Read the model definition and answer for the solid it produces. Units are mm, in the model's axes. Coordinates: 2 decimals unless noted, no trailing zeros. Loops run counter-clockwise (first coordinate to the right, second up) from the corner with the lowest first, then second, coordinate; pieces in that order, holes last. Notation, with made-up numbers: (80.25, 54.25) -> (133.25, 54.25) arc R17 cw to (133.25, 63.25) -> close; hole circle Ø11 at (-29, 83). An arc over 180 degrees is marked (long way). Answer as a JSON object with one key per item and string values. Group by question number.
Q1. This flat-tipped pin is pushed along its axis until it touches: P1, Ø5.5, axis at x = 0, z = -10, coming from the -Y side. Where does it stop, or does it pass through?
Q2. Determine the mould class of faces 1 (the flat face through (-6, -42, 8)), 2 (the cylindrical face through (0.08, -49.82, 1.63)), 3 (the cylindrical face through (-5.43, -43.1, -14.4)), 4 (the cylindrical face through (-5.43, -43.1, 29.4)) for opening direction Z: released by +Z, released by -Z, zero draft, split by the parting line, or undercut.
Q3. The part is cut by section C-C on x = 0. Write down the section's boundary in (y, z).
Q4. The part is cut by section A-A on y = -42.5. Write down the section's boundary in (x, z).
Q5. The part is cut by section D-D on y = -66. Write down the section's boundary in (x, z), and give its area (3 significant figures).
Q6. Straight lines are drawn through the part: line 1 along Z through (x, y) = (-4, -43); line 2 along Y through (x, z) = (0.5, 0); line 3 along X through (y, z) = (-50, -10). For each, find the intervals that lie inside material, in ascending order. Write a range as [from, to].
Q7. The part is cut by section B-B on z = -10. Write down the section's boundary in (x, y), and give its area (3 significant figures).
from build123d import *

# Parameters (mm, degrees)
SKETCH1_W                   = 12
SKETCH1_H                   = 45
BOSS_EXTRUDE1_DEPTH         = 85
TAP_DRILL_FOR_M5X0_8_TAP1_D = 4.2
CUT_EXTRUDE1_REACH          = 92.934
SKETCH3_R                   = 7.5
FILLET1_R                   = 2


with BuildPart() as part:
    # Sketch1 → Boss-Extrude1 (new body)
    with BuildSketch(Plane(origin=(0, 0, 0), x_dir=(1, 0, 0), z_dir=(0, 1, 0))):
        with Locations((0, -7.5)):
            Rectangle(SKETCH1_W, SKETCH1_H)
    extrude(amount=-BOSS_EXTRUDE1_DEPTH)

    # Tap Drill for M5x0.8 Tap1 (through all)
    with Locations(Plane(origin=(0, 0, -10), x_dir=(0, 0, 1), z_dir=(0, 1, 0))):
        with Locations((0, 0), (20, 0), (35, 0)):
            Hole(TAP_DRILL_FOR_M5X0_8_TAP1_D / 2)

    # Sketch3 → Cut-Extrude1 (cut, up to next)
    with BuildSketch(Plane(origin=(6, 0, 0), x_dir=(0, 0, -1), z_dir=(1, 0, 0)), mode=Mode.PRIVATE) as cut_extrude1_sk1:
        with Locations((0, -42.5)):
            Circle(SKETCH3_R)
    cut_extrude1_tool1 = extrude(cut_extrude1_sk1.sketch, amount=-CUT_EXTRUDE1_REACH, mode=Mode.PRIVATE) & part.part
    add(cut_extrude1_tool1.solids().sort_by_distance((6, -42.5, 0))[0], mode=Mode.SUBTRACT)

    # Fillet1
    fillet1_edges = [part.edges().sort_by_distance(p)[0] for p in [
        (6, -42.5, 30),
        (-6, -42.5, 30),
        (-6, -42.5, -15),
        (6, -42.5, -15),
    ]]
    fillet(fillet1_edges, radius=FILLET1_R)


solid = part.part
Final values:
{
 "1": {"P1": "stops at y = -85"},
 "2": {"face 1": "zero draft", "face 2": "undercut", "face 3": "released by -Z", "face 4": "released by +Z"},
 "3": {"outline": "(-85, -15) -> (0, -15) -> (0, -12.1) -> (-85, -12.1) -> close; (-85, -7.9) -> (0, -7.9) -> (0, 7.9) -> (-85, 7.9) -> close; (-85, 12.1) -> (0, 12.1) -> (0, 22.9) -> (-85, 22.9) -> close; (-85, 27.1) -> (0, 27.1) -> (0, 30) -> (-85, 30) -> close; hole circle Ø15 at (-42.5, 0)"},
 "4": {"outline": "(-6, -13) arc R2 ccw to (-4, -15) -> (4, -15) arc R2 ccw to (6, -13) -> (6, -7.5) -> (-6, -7.5) -> close; (-6, 7.5) -> (6, 7.5) -> (6, 28) arc R2 ccw to (4, 30) -> (-4, 30) arc R2 ccw to (-6, 28) -> close; hole circle Ø4.2 at (0, -10); hole circle Ø4.2 at (0, 10); hole circle Ø4.2 at (0, 25)"},
 "5": {"outline": "(-6, -13) arc R2 ccw to (-4, -15) -> (4, -15) arc R2 ccw to (6, -13) -> (6, 28) arc R2 ccw to (4, 30) -> (-4, 30) arc R2 ccw to (-6, 28) -> close; hole circle Ø4.2 at (0, -10); hole circle Ø4.2 at (0, 10); hole circle Ø4.2 at (0, 25)", "area": "495 mm2"},
 "6": {"line 1": "z = [-15, -7.48], [7.48, 30]", "line 2": "y = [-85, -50], [-35, 0]", "line 3": "x = [-6, -2.1], [2.1, 6]"},
 "7": {"outline": "(-6, -85) -> (-2.1, -85) -> (-2.1, 0) -> (-6, 0) -> close; (2.1, -85) -> (6, -85) -> (6, 0) -> (2.1, 0) -> close", "area": "663 mm2"}
}
